Model file for the job. Use its own axes, mm. Face numbers are marked on the shaded views. A direction names the side the tool comes from. Coordinates: 2 decimals unless noted, no trailing zeros. Write each loop counter-clockwise with the first axis right and the second up, starting at its lowest first coordinate (ties: lowest second). Pieces come first, ordered by that corner, then holes.
Q1. Pin check, flat tips, straight feed: P1, Ø2, axis at x = -9.5, y = -3, coming from the -Z side; P2, Ø0.8, axis at y = -12, z = -1.5, coming from the -X side; P3, Ø0.8, axis at x = 4, z = -1, coming from the +Y side. Stop position of each tip, or through.
Q2. Band-saw the part on A-A, the plane x = -2.75. Write the cut outline in (y, z).
Q3. Which spindle directions (+Z, -Z, +X, -X, +Y, -Y) get a long thin tool onto all of the face, cutting with end or side? Do the marked faces 1, 2 and 3. Say none if no direction does.
Q4. Drill centre lines: probe 1 along X at (y, z) = (6, 1.25); probe 2 along Z at (x, y) = (5.5, -0.5); probe 3 along Y at (x, z) = (-0.5, 3.5). Where is each one in solid material? Low to high.
Q5. Band-saw the part on C-C, the plane z = 3. Write the cut outline in (x, y).
Q6. Band-saw the part on B-B, the plane y = 3.25. Write the cut outline in (x, z), plus the area to 3 significant figures.
Q7. Band-saw the part on D-D, the plane y = 5.75. Write the cut outline in (x, z), plus the area to 3 significant figures.
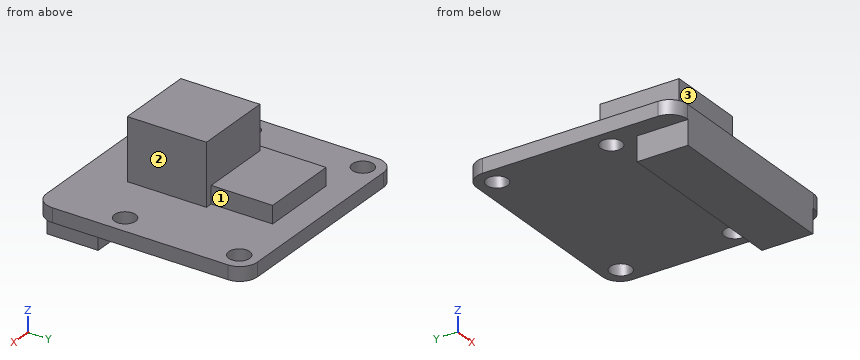
Autodesk Inventor part; units mm, degrees
ref_plane "YZ Plane" through (0, 0, 0) normal (1, 0, 0) x (0, 1, 0)
ref_plane "XZ Plane" through (0, 0, 0) normal (0, 1, 0) x (-1, 0, 0)
ref_plane "XY Plane" through (0, 0, 0) normal (0, 0, 1) x (1, 0, 0)
sketch "Sketch2" plane through (0, 0, 0) normal (0, 0, 1) x (1, 0, 0)
  line L0 (-10.0737, 8.3897) -> (11.1263, 8.3897)
  line L1 (13.1263, 6.3897) -> (13.1263, -13.6103)
  line L2 (11.1263, -15.6103) -> (-10.0737, -15.6103)
  line L3 (-12.0737, -13.6103) -> (-12.0737, 6.3897)
  arc A0 (-10.0737, 8.3897) -> (-12.0737, 6.3897) centre (-10.0737, 6.3897) ccw
  arc A1 (13.1263, 6.3897) -> (11.1263, 8.3897) centre (11.1263, 6.3897) ccw
  arc A2 (11.1263, -15.6103) -> (13.1263, -13.6103) centre (11.1263, -13.6103) ccw
  arc A3 (-12.0737, -13.6103) -> (-10.0737, -15.6103) centre (-10.0737, -13.6103) ccw
  point P0 (0, 0)
  point P1 (-12.0737, 8.3897)
  point P2 (13.1263, -15.6103)
  point P3 (13.1263, 8.3897)
  point P4 (-12.0737, -15.6103)
  dimension "d0" = 25.2
  dimension "d1" = 24
  dimension "d4" = 2
extrude "Extrusion1" add sketch "Sketch2" along normal blind 1.6
sketch "Sketch3" plane through (0, 0, 1.6) normal (0, 0, 1) x (1, 0, 0)
  circle A0 centre (-9.8737, 6.1897) radius 1.2
  circle A1 centre (10.9263, 6.1897) radius 1.2
  circle A2 centre (10.9263, -6.8103) radius 1.2
  circle A3 centre (-9.8737, -6.8103) radius 1.2
  line L0 (11.1263, 8.3897) -> (-10.0737, 8.3897)
  line L1 (-12.0737, 6.3897) -> (-12.0737, -13.6103)
  line L2 (13.1263, -13.6103) -> (13.1263, 6.3897)
  point P0 (0, 0)
  dimension "d5" = 2.4
  dimension "d6" = 2.4
  dimension "d7" = 2.4
  dimension "d8" = 2.4
  dimension "d9" = 2.2
  dimension "d10" = 2.2
  dimension "d11" = 2.2
  dimension "d12" = 2.2
  dimension "d13" = 2.2
  dimension "d14" = 2.2
  dimension "d15" = 13
  dimension "d16" = 13
extrude "Extrusion2" cut sketch "Sketch3" against normal up to next
sketch "Sketch4" plane through (0, 0, 1.6) normal (0, 0, 1) x (1, 0, 0)
  line L0 (-4.8737, 5.3897) -> (4.1263, 5.3897)
  line L1 (4.1263, 5.3897) -> (4.1263, -2.6103)
  line L2 (4.1263, -2.6103) -> (-4.8737, -2.6103)
  line L3 (-4.8737, -2.6103) -> (-4.8737, 5.3897)
  line L4 (11.1263, 8.3897) -> (-10.0737, 8.3897)
  line L5 (13.1263, -13.6103) -> (13.1263, 6.3897)
  point P0 (0, 0)
  dimension "d19" = 9
  dimension "d20" = 8
  dimension "d21" = 3
  dimension "d22" = 9
extrude "Extrusion3" add sketch "Sketch4" along normal blind 2
sketch "Sketch5" plane through (0, 0, 1.6) normal (0, 0, 1) x (1, 0, 0)
  line L0 (-4.0737, -1.6103) -> (4.9263, -1.6103)
  line L1 (4.9263, -1.6103) -> (4.9263, -10.6103)
  line L2 (4.9263, -10.6103) -> (-4.0737, -10.6103)
  line L3 (-4.0737, -10.6103) -> (-4.0737, -1.6103)
  line L4 (-10.0737, -15.6103) -> (11.1263, -15.6103)
  line L5 (-12.0737, 6.3897) -> (-12.0737, -13.6103)
  point P0 (0, 0)
  dimension "d25" = 9
  dimension "d26" = 9
  dimension "d27" = 5
  dimension "d28" = 8
extrude "Extrusion4" add sketch "Sketch5" along normal blind 7
sketch "Sketch6" plane through (0, 0, 0) normal (0, 0, -1) x (-1, 0, 0)
  line L0 (10.0737, -15.6103) -> (-11.1263, -15.6103)
  line L1 (-11.0263, -15.6103) -> (9.9737, -15.6103)
  line L2 (9.9737, -15.6103) -> (9.9737, -9.8103)
  line L3 (9.9737, -9.8103) -> (-11.0263, -9.8103)
  line L4 (-11.0263, -9.8103) -> (-11.0263, -15.6103)
  line L5 (-13.1263, 6.3897) -> (-13.1263, -13.6103)
  point P0 (0, 0)
  dimension "d31" = 21
  dimension "d32" = 5.8
  dimension "d33" = 2.1
extrude "Extrusion5" add sketch "Sketch6" along normal blind 2.78
equation "\"d6\" = d5"
equation "\"d7\" = d5"
equation "\"d8\" = d5"
equation "\"d10\" = d9"
equation "\"d11\" = d9"
equation "\"d12\" = d9"
equation "\"d13\" = d9"
equation "\"d14\" = d9"
equation "\"d16\" = d15"
equation "\"d33\" = -0.5 * d31 + 0.5 * d0"
properties part number "RasPIcam"
Answer sheet:
1. P1: stops at z = 0
1. P2: stops at x = -9.97
1. P3: stops at y = -9.81
2. outline: (-15.61, -2.78) - (-9.81, -2.78) - (-9.81, 0) - (8.39, 0) - (8.39, 1.6) - (5.39, 1.6) - (5.39, 3.6) - (-1.61, 3.6) - (-1.61, 8.6) - (-10.61, 8.6) - (-10.61, 1.6) - (-15.61, 1.6) - close
3. face 1: +Z, +X, +Y
3. face 2: +Z, +X, +Y, -Y
3. face 3: +Z, +X, -X, -Y
4. probe 1: x = -12.07 to -11.06, -8.69 to 9.74, 12.11 to 13.13
4. probe 2: z = 0 to 1.6
4. probe 3: y = -10.61 to 5.39
5. outline: (-4.87, -2.61) - (-4.07, -2.61) - (-4.07, -10.61) - (4.93, -10.61) - (4.93, -1.61) - (4.13, -1.61) - (4.13, 5.39) - (-4.87, 5.39) - close
6. outline: (-12.07, 0) - (13.13, 0) - (13.13, 1.6) - (4.13, 1.6) - (4.13, 3.6) - (-4.87, 3.6) - (-4.87, 1.6) - (-12.07, 1.6) - close
6. area: 58.3 mm2
7. outline: (-12.07, 0) - (-10.99, 0) - (-10.99, 1.6) - (-12.07, 1.6) - close; (-8.76, 0) - (9.81, 0) - (9.81, 1.6) - (-8.76, 1.6) - close; (12.04, 0) - (13.13, 0) - (13.13, 1.6) - (12.04, 1.6) - close
7. area: 33.2 mm2
